Build history of the part. All positions in model axes, mm. A direction names the side the tool comes from. Coordinates: 2 decimals unless noted, no trailing zeros. Write each loop counter-clockwise with the first axis right and the second up, starting at its lowest first coordinate (ties: lowest second). Pieces come first, ordered by that corner, then holes.
```python
from build123d import *

# Parameters (mm, degrees)
F0_W     = 9
F0_H     = 16.7
F0_H_2   = 6.7
F0_W_2   = 16
F0_H_3   = 5.9
F0_W_3   = 95
F0_W_4   = 8.8775146961
F0_W_5   = 6.5
F0_H_4   = 5.7
F0_R     = 1.85
F0_W_6   = 8.7
F0_W_7   = 13.9
F0_H_5   = 29.4
F0_H_6   = 6.8
F0_H_7   = 41.9
F0_H_8   = 6
F0_H_9   = 17.3
F1_DEPTH = 5


with BuildPart() as f1:
    # F0 (on Top) → F1 (new body)
    with BuildSketch(Plane.XY):
        with BuildLine():
            Line((-77.4, 165.8051506788), (-77.4, 123.8051506788))
            Line((-77.4, 123.8051506788), (-63.8979991994, 123.8051506788))
            ThreePointArc((-63.8979991994, 123.8051506788), (-63.1320508076, 125.5079263165), (-61.4, 126.2051506788))
            Line((-61.4, 126.2051506788), (-61.4, 165.8051506788))
            Line((-61.4, 165.8051506788), (-77.4, 165.8051506788))
        make_face()
        with BuildLine():
            Line((-77.4, 123.8051506788), (-77.4, 107.1051506788))
            Line((-77.4, 107.1051506788), (-61.4, 107.1051506788))
            Line((-61.4, 107.1051506788), (-61.4, 121.2051506788))
            ThreePointArc((-61.4, 121.2051506788), (-63.2027756377, 121.9730998712), (-63.8979991994, 123.8051506788))
            Line((-63.8979991994, 123.8051506788), (-77.4, 123.8051506788))
        make_face()
        with BuildLine():
            Line((-31.8387573481, 165.8051506788), (-61.4, 165.8051506788))
            Line((-61.4, 165.8051506788), (-61.4, 126.2051506788))
            ThreePointArc((-61.4, 126.2051506788), (-59.6679491924, 125.5079263165), (-58.9020008006, 123.8051506788))
            Line((-58.9020008006, 123.8051506788), (31.1020008006, 123.8051506788))
            ThreePointArc((31.1020008006, 123.8051506788), (31.8679491924, 125.5079263165), (33.6, 126.2051506788))
            Line((33.6, 126.2051506788), (33.6, 165.8051506788))
            Line((33.6, 165.8051506788), (-4.8387573481, 165.8051506788))
            Line((-4.8387573481, 165.8051506788), (-4.8387573481, 155.8051506788))
            Line((-4.8387573481, 155.8051506788), (-31.8387573481, 155.8051506788))
            Line((-31.8387573481, 155.8051506788), (-31.8387573481, 165.8051506788))
        make_face()
        with BuildLine():
            Line((-61.4, 121.2051506788), (-61.4, 107.1051506788))
            Line((-61.4, 107.1051506788), (33.6, 107.1051506788))
            Line((33.6, 107.1051506788), (33.6, 121.2051506788))
            ThreePointArc((33.6, 121.2051506788), (31.7972243623, 121.9730998712), (31.1020008006, 123.8051506788))
            Line((31.1020008006, 123.8051506788), (-58.9020008006, 123.8051506788))
            ThreePointArc((-58.9020008006, 123.8051506788), (-58.9005002502, 123.7551606858), (-58.9, 123.7051506788))
            ThreePointArc((-58.9, 123.7051506788), (-59.632233047, 121.9373837258), (-61.4, 121.2051506788))
        make_face()
        with BuildLine():
            Line((33.6, 121.2051506788), (33.6, 107.1051506788))
            Line((33.6, 107.1051506788), (49.6, 107.1051506788))
            Line((49.6, 107.1051506788), (49.6, 123.8051506788))
            Line((49.6, 123.8051506788), (36.0979991994, 123.8051506788))
            ThreePointArc((36.0979991994, 123.8051506788), (36.0994997498, 123.7551606858), (36.1, 123.7051506788))
            ThreePointArc((36.1, 123.7051506788), (35.367766953, 121.9373837258), (33.6, 121.2051506788))
        make_face()
        with Locations((54.1, 115.4551506788)):
            Rectangle(F0_W, F0_H)
        with Locations((-81.9, 115.4551506788)):
            Rectangle(F0_W, F0_H)
        with Locations((-81.9, 97.8551506788)):
            Rectangle(F0_W, F0_H_2)
        with Locations((-69.4, 97.8551506788)):
            Rectangle(F0_W_2, F0_H_2)
        with Locations((-69.4, 104.1551506788)):
            Rectangle(F0_W_2, F0_H_3)
        with Locations((-13.9, 104.1551506788)):
            Rectangle(F0_W_3, F0_H_3)
        with Locations((-13.9, 97.8551506788)):
            Rectangle(F0_W_3, F0_H_2)
        with Locations((41.6, 97.8551506788)):
            Rectangle(F0_W_2, F0_H_2)
        with Locations((41.6, 104.1551506788)):
            Rectangle(F0_W_2, F0_H_3)
        with Locations((54.1, 97.8551506788)):
            Rectangle(F0_W, F0_H_2)
        with BuildLine():
            Line((36.0979991994, 123.8051506788), (49.6, 123.8051506788))
            Line((49.6, 123.8051506788), (49.6, 165.8051506788))
            Line((49.6, 165.8051506788), (33.6, 165.8051506788))
            Line((33.6, 165.8051506788), (33.6, 126.2051506788))
            ThreePointArc((33.6, 126.2051506788), (35.3320508076, 125.5079263165), (36.0979991994, 123.8051506788))
        make_face()
        with Locations((54.1, 169.1551506788)):
            Rectangle(F0_W, F0_H_2)
        Polygon((-77.4, 172.5051506788), (-77.4, 165.8051506788), (-61.4, 165.8051506788), (-31.8387573481, 165.8051506788), (-18.3387573481, 165.8051506788), (-4.8387573481, 165.8051506788), (33.6, 165.8051506788), (49.6, 165.8051506788), (49.6, 172.5051506788), (-8.3387573481, 172.5051506788), (-28.3387573481, 172.5051506788), align=None)
        with Locations((-81.8387573481, 169.1551506788)):
            Rectangle(F0_W_4, F0_H_2)
        Polygon((-77.4, 188.7051506788), (-77.4, 172.5051506788), (-28.3387573481, 172.5051506788), (-8.3387573481, 172.5051506788), (49.6, 172.5051506788), (49.6, 188.7051506788), (43.1, 188.7051506788), (32.9, 188.7051506788), (-60.7, 188.7051506788), (-70.9, 188.7051506788), align=None)
        with Locations((-74.15, 191.5551506788)):
            Rectangle(F0_W_5, F0_H_4)
        Polygon((-60.7, 191.5551506788), (-60.7, 188.7051506788), (32.9, 188.7051506788), (32.9, 191.5551506788), (32.9, 194.4051506788), (-60.7, 194.4051506788), align=None)
        with BuildLine():
            ThreePointArc((-53.35, 191.5551506788), (-55.2, 189.7051506788), (-57.05, 191.5551506788))
            ThreePointArc((-57.05, 191.5551506788), (-55.2, 193.4051506788), (-53.35, 191.5551506788))
        make_face(mode=Mode.SUBTRACT)
        with Locations((27.4, 191.5551506788)):
            Circle(F0_R, mode=Mode.SUBTRACT)
        with Locations((46.35, 191.5551506788)):
            Rectangle(F0_W_5, F0_H_4)
        Polygon((-77.4, 208.7051506788), (-77.4, 194.4051506788), (-70.9, 194.4051506788), (-60.7, 194.4051506788), (32.9, 194.4051506788), (43.1, 194.4051506788), (49.6, 194.4051506788), (49.6, 208.7051506788), (-13.9, 208.7051506788), align=None)
        with BuildLine():
            ThreePointArc((-8.9, 202.9051506788), (-17.4355339059, 199.3696167728), (-13.9, 207.9051506788))
            ThreePointArc((-13.9, 207.9051506788), (-10.3644660941, 206.4406845847), (-8.9, 202.9051506788))
        make_face(mode=Mode.SUBTRACT)
        Polygon((-86.4, 208.7051506788), (-77.4, 208.7051506788), (-77.4, 212.6051506788), (-77.4, 218.3051506788), (-77.4, 223.7051506788), (-86.4, 223.7051506788), align=None)
        with Locations((-73.05, 215.4551506788)):
            Rectangle(F0_W_6, F0_H_4)
        Polygon((-77.4, 212.6051506788), (-77.4, 208.7051506788), (-13.9, 208.7051506788), (-13.9, 212.6051506788), (-27.8, 212.6051506788), (-38, 212.6051506788), (-58.5, 212.6051506788), (-68.7, 212.6051506788), align=None)
        Polygon((-77.4, 223.7051506788), (-77.4, 218.3051506788), (-68.7, 218.3051506788), (-58.5, 218.3051506788), (-38, 218.3051506788), (-27.8, 218.3051506788), (-13.9, 218.3051506788), (-13.9, 223.7051506788), align=None)
        Polygon((-58.5, 215.4551506788), (-58.5, 212.6051506788), (-38, 212.6051506788), (-38, 218.3051506788), (-58.5, 218.3051506788), align=None)
        with BuildLine():
            ThreePointArc((-51.65, 215.4551506788), (-53.5, 213.6051506788), (-55.35, 215.4551506788))
            ThreePointArc((-55.35, 215.4551506788), (-53.5, 217.3051506788), (-51.65, 215.4551506788))
        make_face(mode=Mode.SUBTRACT)
        with Locations((-20.85, 215.4551506788)):
            Rectangle(F0_W_7, F0_H_4)
        with Locations((-6.95, 215.4551506788)):
            Rectangle(F0_W_7, F0_H_4)
        Polygon((-13.9, 212.6051506788), (-13.9, 208.7051506788), (49.6, 208.7051506788), (49.6, 212.6051506788), (40.9, 212.6051506788), (30.7, 212.6051506788), (10.2, 212.6051506788), (0, 212.6051506788), align=None)
        Polygon((-13.9, 223.7051506788), (-13.9, 218.3051506788), (0, 218.3051506788), (10.2, 218.3051506788), (30.7, 218.3051506788), (40.9, 218.3051506788), (49.6, 218.3051506788), (49.6, 223.7051506788), align=None)
        Polygon((10.2, 218.3051506788), (10.2, 212.6051506788), (30.7, 212.6051506788), (30.7, 215.4551506788), (30.7, 218.3051506788), align=None)
        with Locations((25.7, 215.4551506788)):
            Circle(F0_R, mode=Mode.SUBTRACT)
        with Locations((45.25, 215.4551506788)):
            Rectangle(F0_W_6, F0_H_4)
        Polygon((49.6, 212.6051506788), (49.6, 208.7051506788), (58.6, 208.7051506788), (58.6, 223.7051506788), (49.6, 223.7051506788), (49.6, 218.3051506788), align=None)
        with Locations((-13.9, 79.8051506788)):
            Rectangle(F0_W_3, F0_H_5)
        with Locations((-69.4, 79.8051506788)):
            Rectangle(F0_W_2, F0_H_5)
        with Locations((41.6, 79.8051506788)):
            Rectangle(F0_W_2, F0_H_5)
        with Locations((41.6, 61.7051506788)):
            Rectangle(F0_W_2, F0_H_6)
        with Locations((54.1, 61.7051506788)):
            Rectangle(F0_W, F0_H_6)
        with Locations((-69.4, 61.7051506788)):
            Rectangle(F0_W_2, F0_H_6)
        with Locations((-81.9, 61.7051506788)):
            Rectangle(F0_W, F0_H_6)
        with Locations((-69.4, 37.3551506788)):
            Rectangle(F0_W_2, F0_H_7)
        with Locations((-13.9, 37.3551506788)):
            Rectangle(F0_W_3, F0_H_7)
        with Locations((41.6, 37.3551506788)):
            Rectangle(F0_W_2, F0_H_7)
        with Locations((-13.9, 61.7051506788)):
            Rectangle(F0_W_3, F0_H_6)
        with BuildLine():
            Line((-77.4, -13.6948493212), (-77.4, -23.2948493212))
            Line((-77.4, -23.2948493212), (-61.4, -23.2948493212))
            Line((-61.4, -23.2948493212), (-61.4, -18.7948493212))
            ThreePointArc((-61.4, -18.7948493212), (-63.9, -16.2948493212), (-61.4, -13.7948493212))
            Line((-61.4, -13.7948493212), (-61.4, -13.6948493212))
            Line((-61.4, -13.6948493212), (-77.4, -13.6948493212))
        make_face()
        with Locations((-69.4, -10.2948493212)):
            Rectangle(F0_W_2, F0_H_6)
        with Locations((-81.9, -10.2948493212)):
            Rectangle(F0_W, F0_H_6)
        with Locations((-69.4, -3.8948493212)):
            Rectangle(F0_W_2, F0_H_8)
        with Locations((-69.4, 7.7551506788)):
            Rectangle(F0_W_2, F0_H_9)
        with Locations((-81.9, 7.7551506788)):
            Rectangle(F0_W, F0_H_9)
        with Locations((-13.9, 7.7551506788)):
            Rectangle(F0_W_3, F0_H_9)
        with Locations((41.6, 7.7551506788)):
            Rectangle(F0_W_2, F0_H_9)
        with Locations((54.1, 7.7551506788)):
            Rectangle(F0_W, F0_H_9)
        with Locations((-13.9, -3.8948493212)):
            Rectangle(F0_W_3, F0_H_8)
        with Locations((-13.9, -10.2948493212)):
            Rectangle(F0_W_3, F0_H_6)
        with BuildLine():
            Line((-61.4, -18.7948493212), (-61.4, -23.2948493212))
            Line((-61.4, -23.2948493212), (33.6, -23.2948493212))
            Line((33.6, -23.2948493212), (33.6, -18.7948493212))
            ThreePointArc((33.6, -18.7948493212), (31.1, -16.2948493212), (33.6, -13.7948493212))
            Line((33.6, -13.7948493212), (33.6, -13.6948493212))
            Line((33.6, -13.6948493212), (-61.4, -13.6948493212))
            Line((-61.4, -13.6948493212), (-61.4, -13.7948493212))
            ThreePointArc((-61.4, -13.7948493212), (-59.632233047, -14.5270823683), (-58.9, -16.2948493212))
            ThreePointArc((-58.9, -16.2948493212), (-59.632233047, -18.0626162742), (-61.4, -18.7948493212))
        make_face()
        with BuildLine():
            Line((33.6, -18.7948493212), (33.6, -23.2948493212))
            Line((33.6, -23.2948493212), (49.6, -23.2948493212))
            Line((49.6, -23.2948493212), (49.6, -13.6948493212))
            Line((49.6, -13.6948493212), (33.6, -13.6948493212))
            Line((33.6, -13.6948493212), (33.6, -13.7948493212))
            ThreePointArc((33.6, -13.7948493212), (35.367766953, -14.5270823683), (36.1, -16.2948493212))
            ThreePointArc((36.1, -16.2948493212), (35.367766953, -18.0626162742), (33.6, -18.7948493212))
        make_face()
        with Locations((41.6, -10.2948493212)):
            Rectangle(F0_W_2, F0_H_6)
        with Locations((41.6, -3.8948493212)):
            Rectangle(F0_W_2, F0_H_8)
        with Locations((54.1, -10.2948493212)):
            Rectangle(F0_W, F0_H_6)
    extrude(amount=F1_DEPTH)


solid = f1.part
```
1. Saw through at A-A on x = 5. List the corners of the cut face in (y, z).
Computed values:
outline: (-23.29, 0) - (212.61, 0) - (212.61, 5) - (-23.29, 5) - close; (218.31, 0) - (223.71, 0) - (223.71, 5) - (218.31, 5) - close
2. Flat gauge pins, fed straight in: pin 1 (1.5 mm diameter, centred on y = 199, z = 3.5, fed in from -X); pin 2 (9 mm diameter, centred on x = -13.9, y = 202.91, fed in from +Z); pin 3 (2 mm diameter, centred on x = 41, y = 82, fed in from -Z). Where does each tip first touch, or does it go through?
Computed values:
pin 1: stops at x = -77.4
pin 2: passes through
pin 3: stops at z = 0
3. Saw through at C-C on z = 1. State how many separate pieces and enclosed holes the cut face has, plus the area to 3 significant figures.
Computed values:
separate pieces: 1
enclosed holes: 16
area: 31,900 mm2
4. Probe line 1 along X through (y, z) = (193.5, 2.2); line 2 along Y through (x, z) = (40, 4.45); line 3 along Y through (x, z) = (-6.5, 1.95). List the from-to ranges inside material, lowest first.
Computed values:
line 1: x = -77.4 to -70.9, -60.7 to 32.9, 43.1 to 49.6
line 2: y = -23.29 to 188.71, 194.41 to 212.61, 218.31 to 223.71
line 3: y = -23.29 to 155.81, 165.81 to 223.71
5. Saw through at B-B on y = 176. List the corners of the cut face in (x, z).
Computed values:
outline: (-77.4, 0) - (49.6, 0) - (49.6, 5) - (-77.4, 5) - close
6. 3-axis set-ups, long thin cutter, end or side, ignore diameter. For faces 1 (the face through (58.6, 8, 2)), 2 (the face through (-82, 165.805, 2)), 3 (the face through (36, 212.605, 2)), 4 (the face through (54, 65.105, 2)): which of +Z, -Z, +X, -X, +Y, -Y reach the whole face in a straight line?
Computed values:
face 1: +Z, -Z, +X, +Y, -Y
face 2: +Z, -Z, -X
face 3: +Z, -Z
face 4: +Z, -Z, +X
7. Mould opens along Y. For faces 5 (the face through (-86.4, 98, 2)), 6 (the face through (49.6, -4, 2)) say: +Y half, -Y half, draft (parallel to the pull), parting line (faces both ways), or undercut.
Computed values:
face 5: draft
face 6: undercut
